Could you check a few things on this model? Use its own coordinates, in mm. A direction names the side the tool comes from. Coordinates: 2 decimals unless noted, no trailing zeros. Order: outer loops, then holes, each group sorted by start corner. A loop starts at its lowest first (then second) coordinate and runs counter-clockwise, first axis right, second up. Notation, with made-up numbers: (68.5, 5.25) - (77.5, 5.25) arc R24 cw to (77.5, 42.25) - close; hole circle Ø5 at (-10, 12). An arc over 180 degrees is marked (long way). Answer as CSV lines item,"result". Start each with the question number.
1. I want a section at C-C, the plane y = -5.25. List the corners of the cut face in (x, z) for me.
2. For faces 1 (the face through (18, -5.6, 12.2)), 2 (the face through (20, 8, 5)), 3 (the face through (9, -1, 5)), which set-ups out of +Z, -Z, +X, -X, +Y, -Y let a thin tool reach every point of the face, with its end or its side?
3. I want a section at B-B, the plane x = 10.5. List the corners of the cut face in (y, z) for me.
4. I want a section at D-D, the plane y = 11.5. List the corners of the cut face in (x, z) for me, and give its area (3 significant figures).
5. I want a section at A-A, the plane z = 2.75. List the corners of the cut face in (x, y) for me, and give its area (3 significant figures).
6. For pin 1 (8 mm diameter, centred on x = 14.5, y = 9, fed in from -Z); pin 2 (2.5 mm diameter, centred on y = -7.5, z = 12, fed in from +X); pin 3 (1.5 mm diameter, centred on x = 20, y = 3, fed in from +Z); pin 4 (3 mm diameter, centred on x = 12.5, z = 4, fed in from +Y), each with a flat end and sliding along its axis, tell me the tip position at first contact or that it passes through.
7. I need wall thicknesses on probe 1 along X at (y, z) = (2, 6.5); probe 2 along Z at (x, y) = (3.25, -4.5); probe 3 along Y at (x, z) = (10, 8.5). Which ranges of each line are inside material? Lowest first, please.
from build123d import *

# Parameters (mm, degrees)
SM_BASE_FLANGE_1_DEPTH      = 10
SM_EDGE_FLANGE_2_DEPTH      = 18
SM_START                    = 1
SM_EDGE_FLANGE_2_FLAT_DEPTH = 1


# Sheet-metal steps are written as plain solids
with BuildPart() as part:
    # Sketch 1 → 基体-法兰1 (new body)
    with BuildSketch(Plane.XY):
        with BuildLine():
            Line((0, 0), (18, 0))
            ThreePointArc((18, 0), (19.414213562, 0.585786438), (20, 2))
            Line((20, 2), (20, 15))
            Line((20, 15), (21, 15))
            Line((21, 15), (21, 2))
            ThreePointArc((21, 2), (20.121320344, -0.121320344), (18, -1))
            Line((18, -1), (0, -1))
            Line((0, -1), (0, 0))
        make_face()
    extrude(amount=SM_BASE_FLANGE_1_DEPTH)

    # 边线-法兰2 bend section (across the edge) → 边线-法兰2 (add)
    with BuildSketch(Plane(origin=(18, -1, 12), x_dir=(0, 0, -1), z_dir=(-1, 0, 0))):
        with BuildLine():
            Line((-1, 2), (0, 2))
            ThreePointArc((0, 2), (0.585786438, 0.585786438), (2, 0))
            Line((2, 0), (2, -1))
            ThreePointArc((2, -1), (-0.121320344, -0.121320344), (-1, 2))
        make_face()
    extrude(amount=SM_EDGE_FLANGE_2_DEPTH)

    # 边线-法兰2 profile (on flange) → 边线-法兰2 flat (add)
    with BuildSketch(Plane(origin=(0, -1, 12), x_dir=(-1, 0, 0), z_dir=(0, 0, 1)).offset(SM_START)):
        Polygon((0, 2), (0, 10), (-1.8, 12.5), (-16.2, 12.5), (-18, 10), (-18, 2), align=None)
    extrude(amount=-SM_EDGE_FLANGE_2_FLAT_DEPTH)


solid = part.part
Solved:
1,outline,"(0, 12) - (18, 12) - (18, 13) - (0, 13) - close"
2,face 1,"+Z, +X, +Y, -Y"
2,face 2,"+Z, -Z, -X, +Y"
2,face 3,"-Z, +X, -X, -Y"
3,outline,"(-13.5, 12) - (-3, 12) arc R2 cw to (-1, 10) - (-1, 0) - (0, 0) - (0, 10) arc R3 ccw to (-3, 13) - (-13.5, 13) - close"
4,outline,"(20, 0) - (21, 0) - (21, 10) - (20, 10) - close"
4,area,"10.0 mm2"
5,outline,"(0, -1) - (18, -1) arc R3 ccw to (21, 2) - (21, 15) - (20, 15) - (20, 2) arc R2 cw to (18, 0) - (0, 0) - close"
5,area,"34.9 mm2"
6,pin 1,"passes through"
6,pin 2,"stops at x = 18"
6,pin 3,"stops at z = 10"
6,pin 4,"stops at y = 0"
7,probe 1,"x = 20 to 21"
7,probe 2,"z = 12 to 13"
7,probe 3,"y = -1 to 0"
